from build123d import *

# Parameters (mm, degrees)
SKETCH1_W               = 44.45
SKETCH1_H               = 44.45
SKETCH1_W_2             = 38.1
SKETCH1_H_2             = 38.1
BOSS_EXTRUDE1_DEPTH     = 1219.2
CUT_EXTRUDE1_DEPTH      = 45.45
F_1_4_CLEARANCE_HOLE1_D = 6.7564
CUT_EXTRUDE2_DEPTH      = 45.45


with BuildPart() as part:
    # Sketch1 → Boss-Extrude1 (new body)
    with BuildSketch(Plane(origin=(0, 0, 0), x_dir=(0, 0, -1), z_dir=(1, 0, 0))):
        with Locations((22.225, 22.225)):
            Rectangle(SKETCH1_W, SKETCH1_H)
        with Locations((22.225, 22.225)):
            Rectangle(SKETCH1_W_2, SKETCH1_H_2, mode=Mode.SUBTRACT)
    extrude(amount=BOSS_EXTRUDE1_DEPTH)

    # Sketch2 → Cut-Extrude1 (cut, through all)
    with BuildSketch(Plane(origin=(0, 44.45, 0), x_dir=(1, 0, 0), z_dir=(0, 1, 0))):
        Polygon((1219.2, 0), (1097.074628705, 44.45), (1219.2, 44.45), align=None)
    extrude(amount=-CUT_EXTRUDE1_DEPTH, mode=Mode.SUBTRACT)

    # 1/4 Clearance Hole1 (through all)
    with Locations(Plane.XY):
        with Locations((39.37, 22.225)):
            Hole(F_1_4_CLEARANCE_HOLE1_D / 2)

    # Sketch5 → Cut-Extrude2 (cut, through all)
    with BuildSketch(Plane(origin=(0, 44.45, 0), x_dir=(1, 0, 0), z_dir=(0, 1, 0))):
        Polygon((1219.2, 0), (1206.5, 0), (1206.5, 4.622421975), align=None)
    extrude(amount=-CUT_EXTRUDE2_DEPTH, mode=Mode.SUBTRACT)


solid = part.part
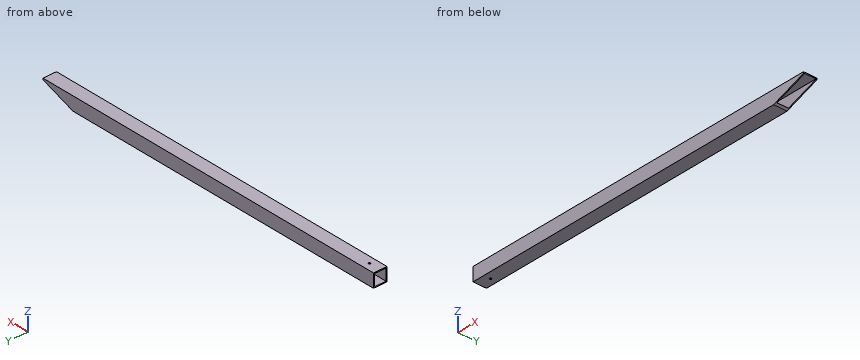
CAD build for the part. Positions are in the model's coordinates, mm. Coordinates: 2 decimals unless noted, no trailing zeros. Order: outer loops, then holes, each group sorted by start corner. A loop starts at its lowest first (then second) coordinate and runs counter-clockwise, first axis right, second up.
Item 1: Band-saw the part on B-B on x = 920. List the corners of the cut face in (y, z) (3 decimals), plus the area to 3 significant figures.
Check sheet entries:
outline: (0, -44.45) - (44.45, -44.45) - (44.45, 0) - (0, 0) - close; hole (3.175, -41.275) - (41.275, -41.275) - (41.275, -3.175) - (3.175, -3.175) - close
area: 524 mm2
Item 2: Band-saw the part on A-A on y = 10. List the corners of the cut face in (x, z) (3 decimals), plus the area to 3 significant figures.
Check sheet entries:
outline: (0, -44.45) - (1097.075, -44.45) - (1105.798, -41.275) - (0, -41.275) - close; (0, -3.175) - (1206.5, -3.175) - (1206.5, 0) - (0, 0) - close
area: 7,330 mm2
Item 3: Drill centre lines: L1, parallel to Z at x = 510.5, y = 26 (3 decimals); L2, parallel to Y at x = 756, z = -37.5 (3 decimals); L3, parallel to Y at x = 39.37, z = -42.1. Where is each one in solid material? Low to high.
Check sheet entries:
L1: z = -44.45 to -41.275, -3.175 to 0
L2: y = 0 to 3.175, 41.275 to 44.45
L3: y = 0 to 18.85, 25.6 to 44.45
